from build123d import *

# Parameters (mm, degrees)
ESQUISSE1_W             = 14.1
ESQUISSE1_H             = 13.1
ESQUISSE1_R             = 1.475
ESQUISSE1_R_2           = 0.4
BOSS_EXTRU_1_DEPTH      = 1.6
ESQUISSE2_W             = 5.75
ESQUISSE2_H             = 7.5
BOSS_EXTRU_2_DEPTH      = 2.45
ENL_V_MAT_EXTRU_1_DEPTH = 5.75
CONG_1_R                = 0.3
ENL_V_MAT_EXTRU_2_DEPTH = 4.5
ESQUISSE5_W             = 3.5
ESQUISSE5_H             = 0.6
BOSS_EXTRU_3_DEPTH      = 3.7


with BuildPart() as part:
    # Esquisse1 → Boss.-Extru.1 (new body)
    with BuildSketch(Plane(origin=(0, 0, 0), x_dir=(1, 0, 0), z_dir=(0, 1, 0))):
        Rectangle(ESQUISSE1_W, ESQUISSE1_H)
        with Locations(Location((-0.175, -4.375, 0), (0, 0, 270))):
            Circle(ESQUISSE1_R, mode=Mode.SUBTRACT)
        with Locations(Location((-0.175, 4.575, 0), (0, 0, 270))):
            Circle(ESQUISSE1_R, mode=Mode.SUBTRACT)
        with Locations(Location((6.178751871, -5.15, 0), (0, 0, 270))):
            Circle(ESQUISSE1_R_2, mode=Mode.SUBTRACT)
        with Locations(Location((6.178751871, -2.575, 0), (0, 0, 270))):
            Circle(ESQUISSE1_R_2, mode=Mode.SUBTRACT)
        with Locations(Location((6.178751871, 0, 0), (0, 0, 270))):
            Circle(ESQUISSE1_R_2, mode=Mode.SUBTRACT)
        with Locations(Location((6.178751871, 2.575, 0), (0, 0, 270))):
            Circle(ESQUISSE1_R_2, mode=Mode.SUBTRACT)
        with Locations(Location((6.178751871, 5.15, 0), (0, 0, 270))):
            Circle(ESQUISSE1_R_2, mode=Mode.SUBTRACT)
    extrude(amount=BOSS_EXTRU_1_DEPTH)

    # Esquisse2 → Boss.-Extru.2 (add)
    with BuildSketch(Plane(origin=(0, 1.6, 0), x_dir=(1, 0, 0), z_dir=(0, 1, 0))):
        with Locations((-4.375, 0)):
            Rectangle(ESQUISSE2_W, ESQUISSE2_H)
    extrude(amount=BOSS_EXTRU_2_DEPTH)

    # Esquisse3 → Enlèv. mat.-Extru.1 (cut)
    with BuildSketch(Plane.ZY.offset(7.25)):
        Polygon((-3.75, 1.6), (-2.95, 1.6), (-3.75, 2.4), align=None)
        Polygon((2.95, 1.6), (3.75, 1.6), (3.75, 2.4), align=None)
    extrude(amount=-ENL_V_MAT_EXTRU_1_DEPTH, mode=Mode.SUBTRACT)

    # Congé1
    cong_1_edges = [part.edges().sort_by_distance(p)[0] for p in [
        (-1.5, 2, 3.35),
        (-1.5, 3.225, 3.75),
        (-1.5, 2, -3.35),
        (-1.5, 3.225, -3.75),
        (-1.5, 4.05, 0),
        (-7.15, 1.6, 2.95),
        (-7.15, 1.6, -2.95),
        (-4.375, 2.4, -3.75),
        (-4.375, 2.4, 3.75),
        (-4.375, 4.05, -3.75),
        (-4.375, 4.05, 3.75),
    ]]
    fillet(cong_1_edges, radius=CONG_1_R)

    # Esquisse4 → Enlèv. mat.-Extru.2 (cut)
    with BuildSketch(Plane.ZY.offset(7.25)):
        Polygon((-3.53, 3.83), (-3.53, 2.491126984), (-2.858873016, 1.82), (2.858873016, 1.82), (3.53, 2.491126984), (3.53, 3.83), align=None)
    extrude(amount=-ENL_V_MAT_EXTRU_2_DEPTH, mode=Mode.SUBTRACT)

    # Esquisse5 → Boss.-Extru.3 (add)
    with BuildSketch(Plane.ZY.offset(2.75)):
        with Locations((0, 2.83)):
            Rectangle(ESQUISSE5_W, ESQUISSE5_H)
    extrude(amount=BOSS_EXTRU_3_DEPTH)


solid = part.part
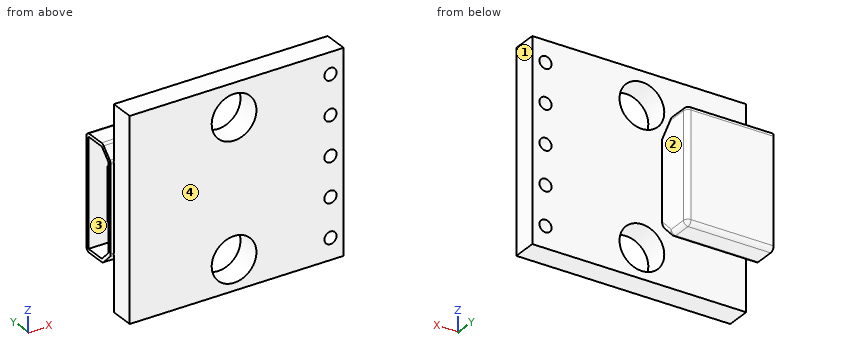
Design review of the part built by this model. Coordinates are the model's own, in mm. Face numbers are marked on the shaded views. A direction names the side the tool comes from. Give positions to 0.01 mm unless a question says otherwise; leave off trailing zeros. Order: outer loops, then holes, each group sorted by start corner. A loop starts at its lowest first (then second) coordinate and runs counter-clockwise, first axis right, second up. Notation, with made-up numbers: (-31.75, -1.75) - (12.25, -1.75) arc R13 cw to (12.25, 12.25) - close; hole circle Ø7 at (7, 62). An arc over 180 degrees is marked (long way). Write item = value, one per line. Start each with the question number.
Q1. We need section B-B on z = 5.15. State the section outline as (x, y) points, plus the area to 3 significant figures.
Q2. Mouldability with a two-part tool opening along Z and no side actions: class the marked faces 3 and 4 as released by +Z, released by -Z, zero draft, split by the parting line, or undercut.
Q3. To check wall thickness, follow L1, parallel to Z at x = -5, y = 2.6; L2, parallel to Y at x = -4.25, z = 1.5; L3, parallel to X at y = 1.1, z = 0. State the ranges of each line that lie inside material, in increasing order. Write a range as from..to.
Q4. Clearance check with flat-ended pins moving along their axes: pin 1 Ø4 at (x, z) = (2, 1) entering from +Y; pin 2 Ø0.5 at (x, y) = (-4.5, 3) entering from -Z; pin 3 Ø1.9 at (y, z) = (0.5, -2.5) entering from -X. State where each tip first meets the part, or that it passes through.
Q5. We need section A-A on z = 0. State the section outline as (x, y) points.
Q6. We need section D-D on x = -1. State the section outline as (y, z) points, plus the area to 3 significant figures.
Q7. We need section C-C on x = -3.25. State the section outline as (y, z) points, plus the area to 3 significant figures.
Q8. Tool access review of the marked faces 1 and 2: name each direction out of +Z, -Z, +X, -X, +Y, -Y from which nothing blocks a thin tool from reaching the whole face with its end or side.
Working result:
q1.outline = (-7.05, 0) - (-1.43, 0) - (-1.43, 1.6) - (-7.05, 1.6) - close; (1.08, 0) - (5.78, 0) - (5.78, 1.6) - (1.08, 1.6) - close; (6.58, 0) - (7.05, 0) - (7.05, 1.6) - (6.58, 1.6) - close
q1.area = 17.3 mm²
q2.face_3 = undercut
q2.face_4 = zero draft
q3.L1 = -3.75..-3.53, -1.75..1.75, 3.53..3.75
q3.L2 = 0..1.82, 2.53..3.13, 3.83..4.05
q3.L3 = -7.05..5.78, 6.58..7.05
q4.pin_1 = 1.6
q4.pin_2 = -3.75
q4.pin_3 = -7.05
q5.outline = (-7.25, 1.6) - (-7.05, 1.6) - (-7.05, 0) - (5.78, 0) - (5.78, 1.6) - (-1.5, 1.6) - (-1.5, 3.75) arc R0.3 ccw to (-1.8, 4.05) - (-7.25, 4.05) - (-7.25, 3.83) - (-2.75, 3.83) - (-2.75, 3.13) - (-6.45, 3.13) - (-6.45, 2.53) - (-2.75, 2.53) - (-2.75, 1.82) - (-7.25, 1.82) - close; (6.58, 0) - (7.05, 0) - (7.05, 1.6) - (6.58, 1.6) - close
q6.outline = (0, -6.55) - (1.6, -6.55) - (1.6, -5.8) - (0, -5.8) - close; (0, -3.35) - (1.6, -3.35) - (1.6, 3.15) - (0, 3.15) - close; (0, 5.6) - (1.6, 5.6) - (1.6, 6.55) - (0, 6.55) - close
q6.area = 13.1 mm²
q7.outline = (0, -6.55) - (1.6, -6.55) - (1.6, -2.95) - (2.31, -3.66) arc R0.3 ccw to (2.52, -3.75) - (3.75, -3.75) arc R0.3 ccw to (4.05, -3.45) - (4.05, 3.45) arc R0.3 ccw to (3.75, 3.75) - (2.52, 3.75) arc R0.3 ccw to (2.31, 3.66) - (1.6, 2.95) - (1.6, 6.55) - (0, 6.55) - close; (2.53, -1.75) - (3.13, -1.75) - (3.13, 1.75) - (2.53, 1.75) - close; hole (1.82, -2.86) - (2.49, -3.53) - (3.83, -3.53) - (3.83, 3.53) - (2.49, 3.53) - (1.82, 2.86) - close
q7.area = 27.0 mm²
q8.face_1 = +Z, -Z, +X, +Y, -Y
q8.face_2 = +Z, -Z, +X, +Y
